Input: part model. Units: mm. Frame: model coordinates. Give positions to 0.01 mm unless a question says otherwise; leave off trailing zeros. Order: outer loops, then holes, each group sorted by start corner. A loop starts at its lowest first (then second) coordinate and runs counter-clockwise, first axis right, second up. Notation, with made-up numbers: (7, 28) -> (29, 28) arc R18 ccw to (29, 51) -> close; hole circle Ø10 at (-23, -25). An arc over 180 degrees is marked (long way). Use a Markdown table: item, result. Add a question column.
Autodesk Inventor part; units mm, degrees
ref_plane "YZ Plane" through (0, 0, 0) normal (1, 0, 0) x (0, 1, 0)
ref_plane "XZ Plane" through (0, 0, 0) normal (0, 1, 0) x (-1, 0, 0)
ref_plane "XY Plane" through (0, 0, 0) normal (0, 0, 1) x (1, 0, 0)
sketch "Sketch1" plane through (0, 0, 0) normal (0, 0, 1) x (1, 0, 0)
  line L0 (0, 0) -> (300, 0)
  line L1 (300, 0) -> (300, 16)
  line L2 (300, 16) -> (0, 16)
  line L3 (0, 16) -> (0, 0)
  line L4 (0, 0) -> (22.0483, 0)
  line L5 (10, 0) -> (29.5, 0)
  line L6 (29.5, 0) -> (29.5, -15)
  line L7 (29.5, -15) -> (10, -15)
  line L8 (10, -15) -> (10, 0)
  point P0 (0, 8)
  dimension "d2" = 19.5
  dimension "d3" = 15
  dimension "d4" = 10
  dimension "d5" = 16
  dimension "d8" = 300
extrude "Extrusion1" add sketch "Sketch1" along normal blind 3
sketch "Sketch2" plane through (0, 0, 3) normal (0, 0, 1) x (1, 0, 0)
  line L0 (0, 16) -> (0, 0)
  line L1 (0, 16) -> (0, 36)
  line L2 (300, 0) -> (300, 16)
  line L3 (340, 16) -> (340, 36)
  line L4 (340, 36) -> (0, 36)
  line L5 (300, 16) -> (0, 16)
  line L6 (50, 16) -> (50, 30)
  line L7 (50, 30) -> (210, 30)
  line L8 (210, 30) -> (210, 16)
  line L9 (40, 36) -> (36, 56)
  line L10 (36, 56) -> (42, 56)
  line L11 (42, 56) -> (46, 36)
  circle A0 centre (330, 30) radius 2.1
  circle A1 centre (330, 20.6) radius 2.1
  circle A2 centre (320.6, 30) radius 2.05
  line L12 (340, 16) -> (300, 16)
  circle A3 centre (310.6, 30) radius 2.05
  circle A4 centre (310.6, 20.6) radius 2.05
  dimension "d44" = 20
  dimension "d45" = 160
  dimension "d46" = 50
  dimension "d47" = 14
  dimension "d48" = 20
  dimension "d49" = 6
  dimension "d50" = 4
  dimension "d51" = 40
  dimension "d83" = 4.2
  dimension "d84" = 4.2
  dimension "d85" = 6
  dimension "d86" = 9.4
  dimension "d87" = 10
  dimension "d97" = 4.1
  dimension "d98" = 9.4
  dimension "d99" = 40
  dimension "d103" = 4.1
  dimension "d104" = 4.1
  dimension "d105" = 10
extrude "Extrusion2" add sketch "Sketch2" against normal blind 3 contours L1 L4 L3 L12 L5 L8 L7 L6 | L9 L10 L11 L4
sketch "Sketch3" plane through (0, 0, 3) normal (0, 0, 1) x (1, 0, 0)
  circle A0 centre (16.5, -6.5) radius 2.1
  circle A1 centre (24.5, -7) radius 2.1
  line L0 (29.5, 0) -> (300, 0)
  line L1 (29.5, -15) -> (29.5, 0)
  point P0 (0, 0)
  dimension "d75" = 4.2
  dimension "d76" = 6.5
  dimension "d77" = 4.2
  dimension "d78" = 7
  dimension "d79" = 5
  dimension "d80" = 8
extrude "Extrusion3" cut sketch "Sketch3" against normal blind 3
sketch "Sketch4" plane through (0, 0, 3) normal (0, 0, 1) x (1, 0, 0)
  line L0 (29.5, 0) -> (300, 0)
  circle A0 centre (41, 18) radius 2.6
  line L1 (340, 36) -> (46, 36)
  point P0 (0, 0)
  dimension "d95" = 18
  dimension "d96" = 5.2
  dimension "d100" = 5
extrude "Extrusion4" cut sketch "Sketch4" against normal blind 3
sketch "Sketch5" plane through (0, 0, 3) normal (0, 0, 1) x (1, 0, 0)
  line L0 (29.5, 0) -> (300, 0)
  arc A0 (300, 0) -> (340, 16) centre (300, 58) ccw
  line L1 (300, 0) -> (300, 16)
  line L2 (300, 0) -> (300, 16)
  line L3 (300, 16) -> (340, 16)
  point P0 (0, 0)
extrude "Extrusion5" add sketch "Sketch5" against normal blind 3
properties part number "Middle_bar"
Q1. Section query A-A (z = 1.8). Give the number of separate pieces and of enclosed holes in the cut face, plus the area to 3 significant figures.
Q2. Draft query along Y for faces 1 (the cylindrical face through (321.253, 4.034, 1.521)), 2 (the flat face through (169, 15, 0)). Return one class per face: +Y half, -Y half, draft (parallel to the pull), parting line (faces both ways), or undercut.
Q3. Section query C-C (x = 278.5). Return loops of the section in (y, z), plus the area to 3 significant figures.
Q4. First-contact query: pin 1 (0.9 mm diameter, centred on x = 151, z = 1.5, fed in from -Y); pin 2 (1 mm diameter, centred on y = 40.5, z = 2, fed in from +X); pin 3 (1.5 mm diameter, centred on y = -9, z = 2, fed in from -X); pin 4 (1 mm diameter, centred on y = 1, z = 2.5, fed in from -X). Flat tips, straight axial feed; report the tip coordinate or a pass-through.
Q5. Section query B-B (y = 49.5). Return loops of the section in (x, z).
Q6. Ray query, line 1 (Y direction, x = 182.5, z = 0.55); line 2 (Y direction, x = 310.6, z = 1.5); line 3 (X direction, y = 25, z = 1.9). Return the intervals inside material, ascending.
Solution:
| question | item | result |
|---|---|---|
| 1 | separate pieces | 1 |
| 1 | enclosed holes | 9 |
| 1 | area | 10,100 mm² |
| 2 | face 1 | -Y half |
| 2 | face 2 | draft |
| 3 | outline | (0, 0) -> (36, 0) -> (36, 3) -> (0, 3) -> close |
| 3 | area | 108 mm² |
| 4 | pin 1 | stops at y = 0 |
| 4 | pin 2 | stops at x = 45.2 |
| 4 | pin 3 | stops at x = 10 |
| 4 | pin 4 | stops at x = 0 |
| 5 | outline | (37.3, 0) -> (43.3, 0) -> (43.3, 3) -> (37.3, 3) -> close |
| 6 | line 1 | y = 0 to 16, 30 to 36 |
| 6 | line 2 | y = 0.98 to 18.55, 22.65 to 27.95, 32.05 to 36 |
| 6 | line 3 | x = 0 to 50, 210 to 340 |
